```python
from build123d import *

# Parameters (mm, degrees)
BASE_FLANGE1_DEPTH              = 10
CUT_EXTRUDE1_DEPTH              = 22.737065119
CUT_EXTRUDE1_DEPTH_BACK         = 22.737065119
SKETCH6_W                       = 7
SKETCH6_H                       = 10
FILLET1_R                       = 1
M2X0_4_TAPPED_HOLE1_D           = 1.6
M2X0_4_TAPPED_HOLE1_CSINK_D     = 2.45
M2X0_4_TAPPED_HOLE1_CSINK_ANGLE = 90


# Sheet-metal steps are written as plain solids
with BuildPart() as part:
    # Sketch1 → Base-Flange1 (new, symmetric)
    with BuildSketch(Plane.XY):
        with BuildLine():
            Line((0, 0), (15, 0))
            ThreePointArc((15, 0), (16.147152873, 3.638304089), (13.120614758, 1.315959713))
            Line((13.120614758, 1.315959713), (11.711075827, 0.802929498))
            ThreePointArc((11.711075827, 0.802929498), (17.007517527, 4.867032155), (15, -1.5))
            Line((15, -1.5), (0, -1.5))
            Line((0, -1.5), (0, 0))
        make_face()
    extrude(amount=BASE_FLANGE1_DEPTH, both=True)

    # Sketch6 → Cut-Extrude1 (cut, two sides: drawn at the far end of the back side and taken through both)
    with BuildSketch(Plane(origin=(0, 0, 0), x_dir=(1, 0, 0), z_dir=(0, 1, 0)).offset(-CUT_EXTRUDE1_DEPTH_BACK)):
        with Locations((15, 0)):
            Rectangle(SKETCH6_W, SKETCH6_H)
    extrude(amount=CUT_EXTRUDE1_DEPTH + CUT_EXTRUDE1_DEPTH_BACK, mode=Mode.SUBTRACT)

    # Fillet1
    fillet1_edges = [part.edges().sort_by_distance(p)[0] for p in [
        (0, -0.75, 10),
        (11.5, -0.75, -5),
        (11.5, -0.75, 5),
        (0, -0.75, -10),
    ]]
    fillet(fillet1_edges, radius=FILLET1_R)

    # M2x0.4 Tapped Hole1 (through all)
    with Locations(Plane(origin=(0, 0, 0), x_dir=(1, 0, 0), z_dir=(0, 1, 0))):
        with Locations((5, 6), (5, -6)):
            CounterSinkHole(M2X0_4_TAPPED_HOLE1_D / 2, M2X0_4_TAPPED_HOLE1_CSINK_D / 2, counter_sink_angle=M2X0_4_TAPPED_HOLE1_CSINK_ANGLE)


solid = part.part
```
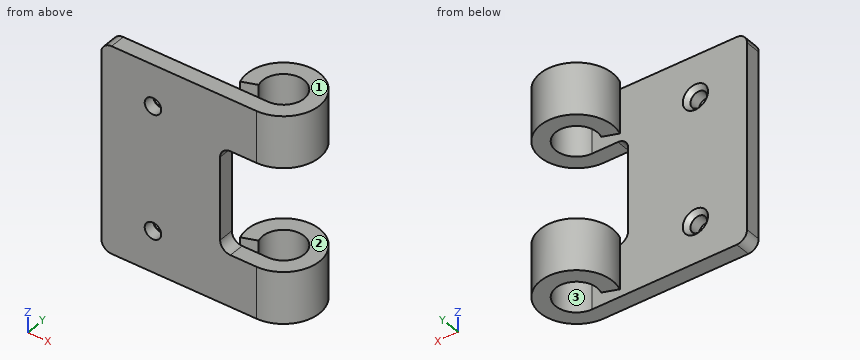
Here's how the part is built. I have some questions about the finished solid (model axes, mm). Face numbers are marked on the shaded views. Coordinates: 2 decimals unless noted, no trailing zeros. Order: outer loops, then holes, each group sorted by start corner. A loop starts at its lowest first (then second) coordinate and runs counter-clockwise, first axis right, second up. Notation, with made-up numbers: (51.25, 25) - (94.25, 25) arc R28 cw to (94.25, 52) - close; hole circle Ø7 at (-36, 12). An arc over 180 degrees is marked (long way). One line per question, with ' | ' between items. Start each with the question number.
1. If we section it at B-B (z = -6): Write out the boundary of the cut face in (x, y) (3 decimals).
2. If we mould it in two halves opening along Z, with no side actions, what happens to the marked faces 1, 2 and 3? For each: released by +Z, released by -Z, zero draft, split by the parting line, or undercut.
3. If we section it at C-C (x = 16): Write out the boundary of the cut face in (y, z).
4. Please list where these lines run through material, in increasing order: line 1 along Z through (x, y) = (5, -0.75); line 2 along Y through (x, z) = (15, -6.85); line 3 along Z through (x, y) = (15, 4.5). Write a range as [from, to].
5. If we section it at A-A (y = 2): Write out the boundary of the cut face in (x, z), and give its area (3 significant figures).
6. If we section it at D-D (x = 5): Write out the boundary of the cut face in (y, z) (3 decimals), and give its area (3 significant figures).
7. I'm going to push flat-ended pins straight in: pin 1 Ø2 at (y, z) = (0, 5.5) entering from +X; pin 2 Ø7.5 at (x, z) = (8.5, -4.5) entering from +Y; pin 3 Ø1.2 at (y, z) = (-1, -0.5) entering from +X. Where does each tip first touch, or does it pass through?
Model answer:
1) outline: (0, -1.5) - (4.2, -1.5) - (4.2, -0.425) - (3.775, 0) - (0, 0) - close; (5.8, -1.5) - (15, -1.5) arc R3.5 ccw (long way) to (11.711, 0.803) - (13.121, 1.316) arc R2 cw (long way) to (15, 0) - (6.225, 0) - (5.8, -0.425) - close
2) face 1: released by +Z | face 2: undercut | face 3: zero draft
3) outline: (-1.35, -10) - (0.27, -10) - (0.27, -5) - (-1.35, -5) - close; (-1.35, 5) - (0.27, 5) - (0.27, 10) - (-1.35, 10) - close; (3.73, -10) - (5.35, -10) - (5.35, -5) - (3.73, -5) - close; (3.73, 5) - (5.35, 5) - (5.35, 10) - (3.73, 10) - close
4) line 1: z = [-10, -6.8], [-5.2, 5.2], [6.8, 10] | line 2: y = [-1.5, 0], [4, 5.5] | line 3: z = [-10, -5], [5, 10]
5) outline: (11.5, -10) - (13, -10) - (13, -5) - (11.5, -5) - close; (11.5, 5) - (13, 5) - (13, 10) - (11.5, 10) - close; (17, -10) - (18.5, -10) - (18.5, -5) - (17, -5) - close; (17, 5) - (18.5, 5) - (18.5, 10) - (17, 10) - close | area: 30.0 mm²
6) outline: (-1.5, -10) - (0, -10) - (0, -7.225) - (-0.425, -6.8) - (-1.5, -6.8) - close; (-1.5, -5.2) - (-0.425, -5.2) - (0, -4.775) - (0, 4.775) - (-0.425, 5.2) - (-1.5, 5.2) - close; (-1.5, 6.8) - (-0.425, 6.8) - (0, 7.225) - (0, 10) - (-1.5, 10) - close | area: 24.8 mm²
7) pin 1: stops at x = 18.35 | pin 2: stops at y = 4.12 | pin 3: stops at x = 11.5
